from build123d import *

# Parameters (mm, degrees)
F1_DEPTH = 10
F2_R     = 1.5
F3_DEPTH = 10.001


with BuildPart() as f1:
    # F0 (on Top) → F1 (new body)
    with BuildSketch(Plane.XY):
        Polygon((13.363348, 15.175648), (-106.636652, 15.175648), (-106.636652, 10.175648), (3.363348, 10.175648), (8.363348, 5.175648), (13.363348, 5.175648), (98.363348, 5.175648), (98.363348, 10.175648), (13.363348, 10.175648), align=None)
    extrude(amount=F1_DEPTH)

    # F2 (on face) → F3 (cut, through all)
    with BuildSketch(Plane.XZ.offset(-5.175648)):
        with Locations((88.363348, 5)):
            Circle(F2_R)
        with Locations((68.363348, 5)):
            Circle(F2_R)
        with Locations((28.363348, 5)):
            Circle(F2_R)
    extrude(amount=-F3_DEPTH, mode=Mode.SUBTRACT)


solid = f1.part
Verification items for the finished model (mm, model axes). A direction names the side the tool comes from. Coordinates: 2 decimals unless noted, no trailing zeros. Order: outer loops, then holes, each group sorted by start corner. A loop starts at its lowest first (then second) coordinate and runs counter-clockwise, first axis right, second up.
Item 1: Section check C-C, the plane x = -6. Enter the section's corners in (y, z).
Filled in:
outline: (10.18, 0) - (15.18, 0) - (15.18, 10) - (10.18, 10) - close
Item 2: Access from +Z, -Z, +X, -X, +Y, -Y to the whole of each face (thin tool, end or side, straight path). Record for faces 1 (the face through (13.363, 13, 5)), 2 (the face through (-52, 10.176, 5)), 3 (the face through (-6, 11, 10)).
Filled in:
face 1: +Z, -Z, +X, +Y
face 2: +Z, -Z, -X, -Y
face 3: +Z, +X, -X, +Y, -Y
Item 3: Section check A-A, the plane z = 5. Enter the section's corners in (x, y).
Filled in:
outline: (-106.64, 10.18) - (3.36, 10.18) - (8.36, 5.18) - (26.86, 5.18) - (26.86, 10.18) - (13.36, 10.18) - (13.36, 15.18) - (-106.64, 15.18) - close; (29.86, 5.18) - (66.86, 5.18) - (66.86, 10.18) - (29.86, 10.18) - close; (69.86, 5.18) - (86.86, 5.18) - (86.86, 10.18) - (69.86, 10.18) - close; (89.86, 5.18) - (98.36, 5.18) - (98.36, 10.18) - (89.86, 10.18) - close
Item 4: Section check B-B, the plane y = 6.75. Enter the section's corners in (x, z).
Filled in:
outline: (6.79, 0) - (98.36, 0) - (98.36, 10) - (6.79, 10) - close; hole circle Ø3 at (28.36, 5); hole circle Ø3 at (68.36, 5); hole circle Ø3 at (88.36, 5)
Item 5: Material ranges on L1, parallel to X at y = 6.25, z = 5.25; L2, parallel to X at y = 7, z = 6; L3, parallel to Y at x = -85, z = 1.75, recorded low to high.
Filled in:
L1: x = 7.29 to 26.88, 29.84 to 66.88, 69.84 to 86.88, 89.84 to 98.36
L2: x = 6.54 to 27.25, 29.48 to 67.25, 69.48 to 87.25, 89.48 to 98.36
L3: y = 10.18 to 15.18
Item 6: Depth check by flat-ended pin: pin 1 (3 mm diameter, centred on x = 42.5, z = 8, fed in from +Y); pin 2 (6 mm diameter, centred on y = 13, z = 2, fed in from +X); pin 3 (4 mm diameter, centred on y = 12.5, z = 5.5, fed in from +X). Enter the tip coordinate at first touch or a pass-through.
Filled in:
pin 1: stops at y = 10.18
pin 2: stops at x = 98.36
pin 3: stops at x = 13.36
